Source: CAD feature listing. Evaluate the final solid. Frame: model axes, mm. Face numbers are marked on the shaded views. A direction names the side the tool comes from. Give positions to 0.01 mm unless a question says otherwise; leave off trailing zeros. Loops run counter-clockwise (first coordinate to the right, second up) from the corner with the lowest first, then second, coordinate; pieces in that order, holes last.
```python
from build123d import *

# Parameters (mm, degrees)
F2_W     = 16.383304
F2_H     = 3.304196
F3_DEPTH = 10
F5_DEPTH = 37.3


with BuildPart() as f1:
    # F0 (on Front) → F1 (revolve)
    with BuildSketch(Plane.XZ):
        Polygon((0, -37.3), (0, 2.7), (-18.25, 2.7), (-18.25, 0), (-14.25, 0), (-14.25, -37.3), align=None)
    revolve(axis=Axis((0, 0, -17.3), (0, 0, 1)))

    # F2 (on face) → F3 (cut)
    with BuildSketch(Plane.XY.offset(2.7)):
        with Locations((0, 6.608392)):
            Rectangle(F2_W, F2_H)
        with Locations((0, -7.159091)):
            Rectangle(F2_W, F2_H)
    extrude(amount=-F3_DEPTH, mode=Mode.SUBTRACT)

    # F4 (on face) → F5 (cut, through all)
    with BuildSketch(Plane(origin=(0, 0, -37.3), x_dir=(1, 0, 0), z_dir=(0, 0, -1))):
        with BuildLine():
            ThreePointArc((5.836309, 13), (0, 14.25), (-5.836309, 13))
            Line((-5.836309, 13), (5.836309, 13))
        make_face()
        with BuildLine():
            Line((5.836309, -13), (-5.836309, -13))
            ThreePointArc((-5.836309, -13), (0, -14.25), (5.836309, -13))
        make_face()
    extrude(amount=-F5_DEPTH, mode=Mode.SUBTRACT)


solid = f1.part
```
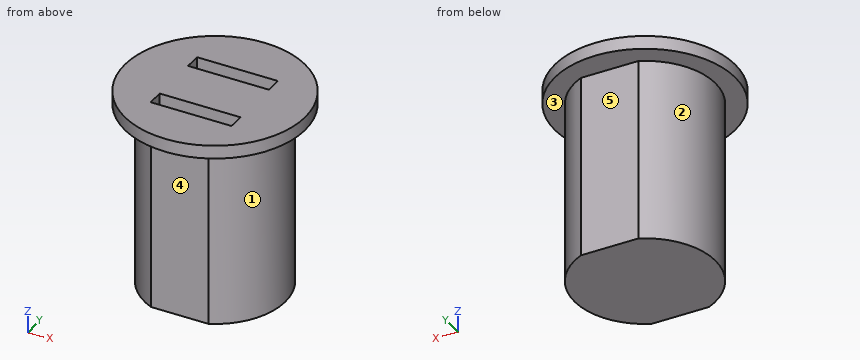
(1) Ray query, line 1 along Y through (x, z) = (-2.5, -4); line 2 along Z through (x, y) = (-8, 6); line 3 along Y through (x, z) = (-5, -20.5). Return the intervals inside material, ascending.
A:
line 1: y = -13 to -8.81, -5.51 to 4.96, 8.26 to 13
line 2: z = -37.3 to -7.3
line 3: y = -13 to 13
(2) Section A-A, the plane x = 0. Return the cut outline in (y, z).
A:
outline: (-18.25, 0) - (-13, 0) - (-13, -37.3) - (13, -37.3) - (13, 0) - (18.25, 0) - (18.25, 2.7) - (8.26, 2.7) - (8.26, -7.3) - (4.96, -7.3) - (4.96, 2.7) - (-5.51, 2.7) - (-5.51, -7.3) - (-8.81, -7.3) - (-8.81, 2.7) - (-18.25, 2.7) - close
(3) Reachability of the marked faces 1, 2, 3, 4 and 5 from +Z, -Z, +X, -X, +Y, -Y: full face, straight path, thin tool, end or side. Return the list, or none.
A:
face 1: -Z, +X
face 2: -Z, -X
face 3: -Z
face 4: -Z, +X, -X, -Y
face 5: -Z, +X, -X, +Y
(4) First-contact query: pin 1 (8 mm diameter, centred on y = 14, z = -30, fed in from -X); pin 2 (1.7 mm diameter, centred on y = 6.5, z = -3, fed in from -X); pin 3 (3 mm diameter, centred on x = 0, z = -2.5, fed in from -Y). Flat tips, straight axial feed; report the tip coordinate or a pass-through.
A:
pin 1: stops at x = -10.15
pin 2: stops at x = -13.08
pin 3: stops at y = -13
(5) Section B-B, the plane y = 0. Return the cut outline in (x, z), then the cut area to 3 significant figures.
A:
outline: (-18.25, 0) - (-14.25, 0) - (-14.25, -37.3) - (14.25, -37.3) - (14.25, 0) - (18.25, 0) - (18.25, 2.7) - (-18.25, 2.7) - close
area: 1,160 mm2
(6) Section C-C, the plane z = -26. Return the cut outline in (x, y), then the cut area to 3 significant figures.
A:
outline: (-5.84, -13) - (5.84, -13) arc R14.25 ccw to (5.84, 13) - (-5.84, 13) arc R14.25 ccw to start
area: 618 mm2
(7) Section D-D, the plane y = 12. Return the cut outline in (x, z).
A:
outline: (-13.75, 0) - (-7.69, 0) - (-7.69, -37.3) - (7.69, -37.3) - (7.69, 0) - (13.75, 0) - (13.75, 2.7) - (-13.75, 2.7) - close
